```python
from build123d import *

# Parameters (mm, degrees)
F0_R     = 22.5
F1_DEPTH = 1.6
F4_D     = 2.75
F2_R     = 2.25
F5_DEPTH = 10
F6_R     = 1.75
F7_R     = 1.75
F8_R     = 1.75
F9_DEPTH = 2


with BuildPart() as f1:
    # F0 (on Front) → F1 (new body)
    with BuildSketch(Plane.XZ):
        Circle(F0_R)
    extrude(amount=F1_DEPTH)

    # F4 (through all)
    with Locations(Plane(origin=(0, 0, 0), x_dir=(-1, 0, 0), z_dir=(0, 1, 0))):
        with Locations((11.821247, 6.825), (0, -13.65), (-11.821247, 6.825)):
            Hole(F4_D / 2)

    # F2 (on face) → F5 (join)
    with BuildSketch(Plane(origin=(0, 0, 0), x_dir=(-1, 0, 0), z_dir=(0, 1, 0))):
        with Locations((0, 14.25)):
            Circle(F2_R)
        with Locations((-12.340862, -7.125)):
            Circle(F2_R)
        with Locations((12.340862, -7.125)):
            Circle(F2_R)
    extrude(amount=-F5_DEPTH)

    # F6 (on face) + F7 (on face) + F8 (on face) → F9 (join)
    with BuildSketch(Plane.XZ.offset(10)):
        with Locations((0, 14.25)):
            Circle(F6_R)
    with BuildSketch(Plane.XZ.offset(10)):
        with Locations((-12.340862, -7.125)):
            Circle(F7_R)
    with BuildSketch(Plane.XZ.offset(10)):
        with Locations((12.340862, -7.125)):
            Circle(F8_R)
    extrude(amount=F9_DEPTH)


solid = f1.part
```
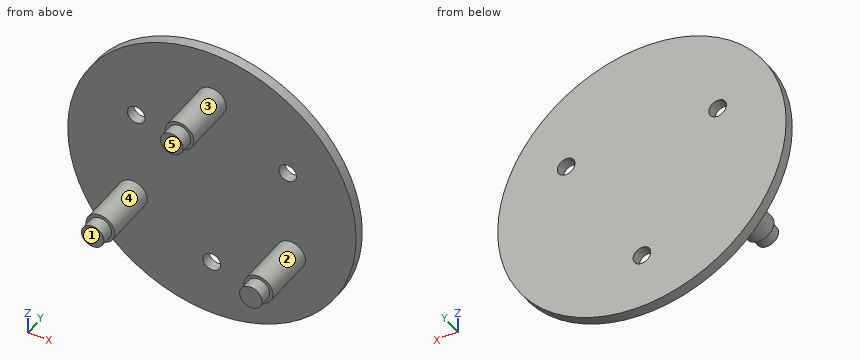
Here's how the part is built. I have some questions about the finished solid (model axes, mm). Face numbers are marked on the shaded views. A direction names the side the tool comes from. Coordinates: 2 decimals unless noted, no trailing zeros. Order: outer loops, then holes, each group sorted by start corner. A loop starts at its lowest first (then second) coordinate and runs counter-clockwise, first axis right, second up. Notation, with made-up numbers: (46, -18.75) - (86, -18.75) arc R13 ccw to (86, 6.25) - close; hole circle Ø6 at (26.25, 3). An arc over 180 degrees is marked (long way). One line per question, with ' | ' between items. Start each with the question number.
1. If we section it at B-B (z = -13.65): Write out the boundary of the cut face in (x, y) (3 decimals).
2. If we section it at D-D (y = -7.75): Write out the boundary of the cut face in (x, z) (3 decimals).
3. If we section it at C-C (z = 14.25): Write out the boundary of the cut face in (x, y).
4. I'm going to push flat-ended pins straight in: pin 1 Ø6 at (x, y) = (16, -4) entering from -Z; pin 2 Ø2 at (x, y) = (13, -7.5) entering from +Z (3 decimals); pin 3 Ø2.5 at (x, z) = (0, -13.65) entering from -Y; pin 4 Ø3 at (x, z) = (17.5, 14) entering from -Y. Where does each tip first touch, or does it pass through?
5. If we mould it in two halves opening along X, with no side actions, what happens to the marked faces 3, 4 and 5? For each: released by +X, released by -X, zero draft, split by the parting line, or undercut.
6. Please list where these lines run through material, in increasing order: line 1 along Z through (x, y) = (0, -1) (3 decimals); line 2 along Z through (x, y) = (12.5, -5); line 3 along Y through (x, z) = (-9.5, -15.5). Write a range as [from, to].
7. If we section it at A-A (x = 0): Write out the boundary of the cut face in (y, z) (3 decimals), and give its area (3 significant figures).
8. Which directions (+Z, -Z, +X, -X, +Y, -Y) give clear straight access to the entire face, cutting with the end or side of a thin tool? Please do the marked faces 1 and 2.
Model answer:
1) outline: (-17.887, -1.6) - (-1.375, -1.6) - (-1.375, 0) - (-17.887, 0) - close; (1.375, -1.6) - (17.887, -1.6) - (17.887, 0) - (1.375, 0) - close
2) outline: circle Ø4.5 at (-12.341, -7.125); circle Ø4.5 at (0, 14.25); circle Ø4.5 at (12.341, -7.125)
3) outline: (-17.41, -1.6) - (-2.25, -1.6) - (-2.25, -10) - (-1.75, -10) - (-1.75, -12) - (1.75, -12) - (1.75, -10) - (2.25, -10) - (2.25, -1.6) - (17.41, -1.6) - (17.41, 0) - (-17.41, 0) - close
4) pin 1: stops at z = -17.45 | pin 2: stops at z = -4.875 | pin 3: passes through | pin 4: stops at y = -1.6
5) face 3: split by the parting line | face 4: undercut | face 5: zero draft
6) line 1: z = [-22.5, -15.025], [-12.275, 22.5] | line 2: z = [-9.37, -4.88] | line 3: y = [-1.6, 0]
7) outline: (-12, 12.5) - (-10, 12.5) - (-10, 12) - (-1.6, 12) - (-1.6, -12.275) - (0, -12.275) - (0, 22.5) - (-1.6, 22.5) - (-1.6, 16.5) - (-10, 16.5) - (-10, 16) - (-12, 16) - close; (-1.6, -22.5) - (0, -22.5) - (0, -15.025) - (-1.6, -15.025) - close | area: 112 mm²
8) face 1: +Z, -Z, +X, -X, -Y | face 2: -Y
